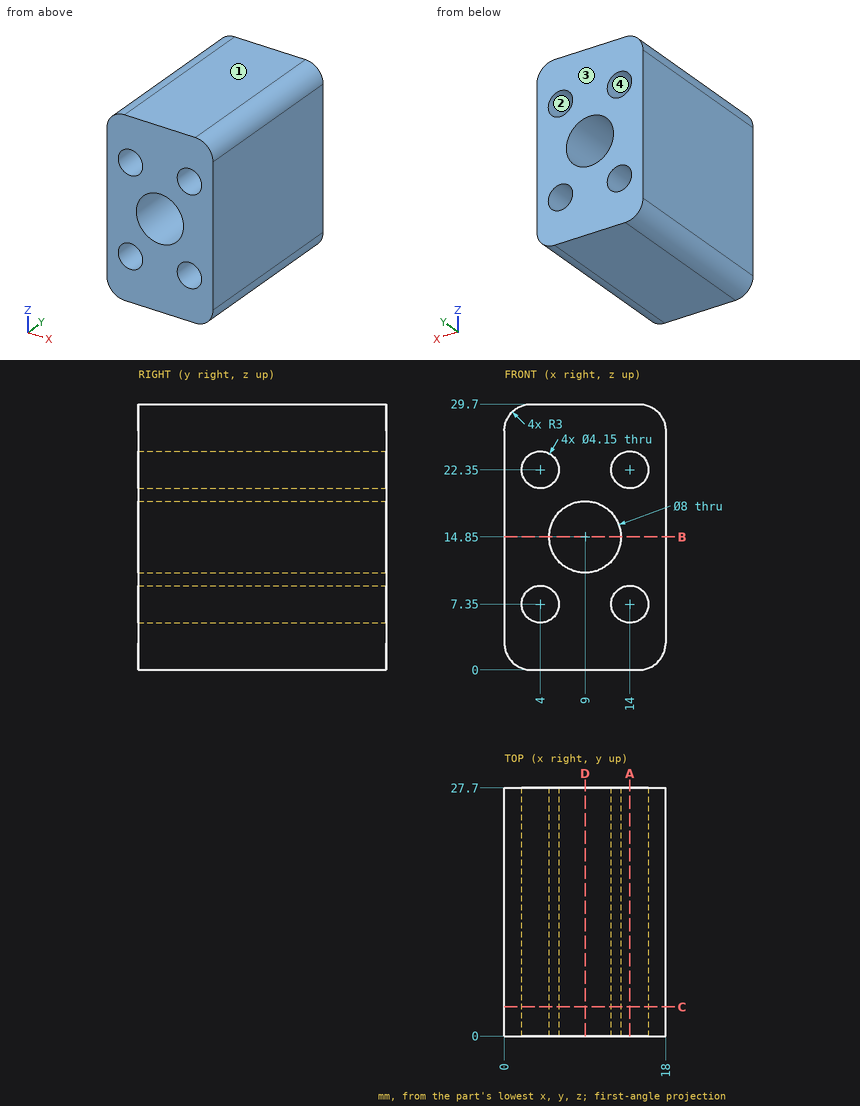
Geometry: see drawing. Coordinates: mm, zero at the bounding-box minimum. Coordinates: 2 decimals unless noted, no trailing zeros. Order: outer loops, then holes, each group sorted by start corner. A loop starts at its lowest first (then second) coordinate and runs counter-clockwise, first axis right, second up. Notation, with made-up numbers: M 44,-15.75 L 64,-15.75 A25 cw 64,2.25 Z; hole C 65.25,21 d5. An arc over 180 degrees is marked long. Answer in a Markdown table with one row per item. Add a question column.
Q1. Section query B-B on z = 14.85. Return the cut outline in (x, y).
Q2. Contact query for a flat-ended pin moving along its axis: P1, Ø1, axis at x = 16, z = 22, coming from the +Y side. Output: stop coordinate, or through.
Q3. Section query D-D on x = 9. Return the cut outline in (y, z).
Q4. Section query C-C on y = 3.25. Return the cut outline in (x, z) (3 decimals), and give its area (3 significant figures).
Q5. Mould query, pull axis Z, two halves, no side actions, for the marked faces 1, 2, 3 and 4. Classes: released by +Z, released by -Z, zero draft, split by the parting line, or undercut.
Q6. Line query: L1, parallel to Z at x = 14, y = 7.5 (3 decimals); L2, parallel to X at y = 9.5, z = 7.35 (3 decimals); L3, parallel to Z at x = 3.25, y = 19. Output: solid intervals per line, ascending.
Q7. Section query A-A on x = 14. Return the cut outline in (y, z) (3 decimals).
Completed:
| question | item | result |
|---|---|---|
| 1 | outline | M 0,0 L 5,0 L 5,27.7 L 0,27.7 Z; M 13,0 L 18,0 L 18,27.7 L 13,27.7 Z |
| 2 | P1 | stops at y = 27.7 |
| 3 | outline | M 0,0 L 27.7,0 L 27.7,10.85 L 0,10.85 Z; M 0,18.85 L 27.7,18.85 L 27.7,29.7 L 0,29.7 Z |
| 4 | outline | M 0,3 A3 ccw 3,0 L 15,0 A3 ccw 18,3 L 18,26.7 A3 ccw 15,29.7 L 3,29.7 A3 ccw 0,26.7 Z; hole C 4,7.35 d4.15; hole C 4,22.35 d4.15; hole C 9,14.85 d8; hole C 14,7.35 d4.15; hole C 14,22.35 d4.15 |
| 4 | area | 423 mm2 |
| 5 | face 1 | released by +Z |
| 5 | face 2 | undercut |
| 5 | face 3 | zero draft |
| 5 | face 4 | undercut |
| 6 | L1 | z = 0 to 5.275, 9.425 to 20.275, 24.425 to 29.7 |
| 6 | L2 | x = 0 to 1.925, 6.075 to 11.925, 16.075 to 18 |
| 6 | L3 | z = 0 to 5.42, 9.28 to 20.42, 24.28 to 29.7 |
| 7 | outline | M 0,0 L 27.7,0 L 27.7,5.275 L 0,5.275 Z; M 0,9.425 L 27.7,9.425 L 27.7,20.275 L 0,20.275 Z; M 0,24.425 L 27.7,24.425 L 27.7,29.7 L 0,29.7 Z |
